Input: part model. Units: mm. Frame: model coordinates. A direction names the side the tool comes from. Coordinates: 2 decimals unless noted, no trailing zeros. Loops run counter-clockwise (first coordinate to the right, second up) from the corner with the lowest first, then second, coordinate; pieces in that order, holes last. Notation, with made-up numbers: (42.5, 51) - (60.5, 51) arc R32 cw to (60.5, 81) - close; hole circle Ø2 at (72.5, 10.5). An arc over 180 degrees is marked (long way). Use a Markdown table: item, result. Add a question column.
1. Draft query along Z for faces 1 (the face through (-55.355, -25, 13)), 2 (the face through (34, -38, 0)), 3 (the face through (-40.033, -25.044, 29.928)). Return one class per face: released by +Z, released by -Z, zero draft, split by the parting line, or undercut.
2. Section query A-A on y = -42. Return the cut outline in (x, z), then the cut area to 3 significant figures.
3. Section query D-D on x = 14. Return the cut outline in (y, z).
4. Access query for faces 4 (the face through (-21, -50.8, 17)), 5 (the face through (21, -25.4, 19)). Directions: +Z, -Z, +X, -X, +Y, -Y. A direction counts if a zero-diameter tool reaches every point of the face in a straight line with its end or side. Return the directions, or none.
5. Section query B-B on z = 46. Return the cut outline in (x, y), then the cut area to 3 significant figures.
6. Section query C-C on x = -28. Return the cut outline in (y, z).
7. Ray query, L1, parallel to Y at x = 26.5, z = 3; L2, parallel to Z at x = -2.5, y = -25.5; L3, parallel to X at y = -39, z = 1. Return the intervals inside material, ascending. Write a range as [from, to].
8. Contact query for flat-ended pins moving along their axis: P1, Ø12, axis at y = -22.5, z = 45.5, coming from the -X side; P2, Ø6, axis at x = -26.5, y = -24.5, coming from the +Z side; P3, Ø4, axis at y = -27.5, z = 15, coming from the +X side. Output: stop coordinate, or through.
```python
from build123d import *

# Parameters (mm, degrees)
F0_R     = 12.7
F1_DEPTH = 25.4
F2_R     = 12.7
F3_DEPTH = 25.4


with BuildPart() as f1:
    # F0 (on Front) → F1 (new body)
    with BuildSketch(Plane.XZ):
        with BuildLine():
            Line((71.645316, -0.444731), (-15.716811, 58.689598))
            ThreePointArc((-15.716811, 58.689598), (-41.860943, 60.091868), (-55.354684, 37.655269))
            Line((-55.354684, 37.655269), (-55.354684, -13.144731))
            Line((-55.354684, -13.144731), (71.645316, -13.144731))
            Line((71.645316, -13.144731), (71.645316, -0.444731))
        make_face()
        with Locations((-29.954684, 37.655269)):
            Circle(F0_R, mode=Mode.SUBTRACT)
    extrude(amount=F1_DEPTH)

    # F2 (on face) → F3 (join)
    with BuildSketch(Plane.XZ.offset(25.4)):
        with BuildLine():
            Line((-4.554684, 0), (-4.554684, 37.655269))
            ThreePointArc((-4.554684, 37.655269), (-7.518084, 49.561528), (-15.716811, 58.689598))
            ThreePointArc((-15.716811, 58.689598), (-41.860943, 60.091868), (-55.354684, 37.655269))
            Line((-55.354684, 37.655269), (-55.354684, 0))
            Line((-55.354684, 0), (-55.354684, -13.144731))
            Line((-55.354684, -13.144731), (71.645316, -13.144731))
            Line((71.645316, -13.144731), (71.645316, -0.444731))
            Line((71.645316, -0.444731), (70.988293, 0))
            Line((70.988293, 0), (-4.554684, 0))
        make_face()
        with Locations((-29.954684, 37.655269)):
            Circle(F2_R, mode=Mode.SUBTRACT)
    extrude(amount=F3_DEPTH)


solid = f1.part
```
Resolved:
| question | item | result |
|---|---|---|
| 1 | face 1 | zero draft |
| 1 | face 2 | released by +Z |
| 1 | face 3 | undercut |
| 2 | outline | (-55.35, -13.14) - (71.65, -13.14) - (71.65, -0.44) - (70.99, 0) - (-4.55, 0) - (-4.55, 37.66) arc R25.4 ccw to (-15.72, 58.69) arc R25.4 ccw to (-55.35, 37.66) - close; hole circle Ø25.4 at (-29.95, 37.66) |
| 2 | area | 4,090 mm² |
| 3 | outline | (-50.8, -13.14) - (0, -13.14) - (0, 38.57) - (-25.4, 38.57) - (-25.4, 0) - (-50.8, 0) - close |
| 4 | face 4 | +Z, -Z, +X, -X, -Y |
| 4 | face 5 | +Z, +X, -Y |
| 5 | outline | (-53.94, -50.8) - (-39.53, -50.8) - (-39.53, 0) - (-53.94, 0) - close; (-20.38, -50.8) - (-5.96, -50.8) - (-5.96, -25.4) - (3.03, -25.4) - (3.03, 0) - (-20.38, 0) - close |
| 5 | area | 1,690 mm² |
| 6 | outline | (-50.8, -13.14) - (0, -13.14) - (0, 25.11) - (-50.8, 25.11) - close; (-50.8, 50.2) - (0, 50.2) - (0, 62.98) - (-50.8, 62.98) - close |
| 7 | L1 | [-25.4, 0] |
| 7 | L2 | [-13.14, 0] |
| 7 | L3 | [-55.35, -4.55] |
| 8 | P1 | x = -55.29 |
| 8 | P2 | z = 63.05 |
| 8 | P3 | x = -4.55 |
